For this review, take the finished solid that the model builds, in its own axes (mm). A direction names the side the tool comes from. Coordinates: 2 decimals unless noted, no trailing zeros. Write each loop counter-clockwise with the first axis right and the second up, starting at its lowest first coordinate (ties: lowest second). Pieces come first, ordered by that corner, then holes.
```python
from build123d import *

# Parameters (mm, degrees)
SKETCH1_W                    = 42.8625
SKETCH1_H                    = 44.27474
SKETCH1_R                    = 3
BASE_FLANGE1_DEPTH           = 3.175
EDGE_FLANGE1_STRIP_W         = 14.7
EDGE_FLANGE1_STRIP_H         = 3.175
EDGE_FLANGE1_STRIP_CUT_DEPTH = 44.27474
EDGE_FLANGE1_DEPTH           = 44.27474
CUT_EXTRUDE1_DEPTH           = 73.0427273
CUT_EXTRUDE1_DEPTH_BACK      = 3.175
M6_CLEARANCE_HOLE6_D         = 7


# Sheet-metal steps are written as plain solids
with BuildPart() as part:
    # Sketch1 → Base-Flange1 (new body)
    with BuildSketch(Plane.XY):
        Rectangle(SKETCH1_W, SKETCH1_H)
        with Locations((-0.79375, 3.26263)):
            Circle(SKETCH1_R, mode=Mode.SUBTRACT)
    extrude(amount=BASE_FLANGE1_DEPTH)

    # Edge-Flange1 strip (across the edge) → Edge-Flange1 strip cut (cut)
    with BuildSketch(Plane(origin=(-21.43125, 22.13737, 3.175), x_dir=(1, 0, 0), z_dir=(0, -1, 0))):
        with Locations((-6.35, -1.5875)):
            Rectangle(EDGE_FLANGE1_STRIP_W, EDGE_FLANGE1_STRIP_H)
    extrude(amount=EDGE_FLANGE1_STRIP_CUT_DEPTH, mode=Mode.SUBTRACT)

    # Edge-Flange1 section (across the edge) → Edge-Flange1 (add)
    with BuildSketch(Plane(origin=(-21.43125, 22.13737, 3.175), x_dir=(1, 0, 0), z_dir=(0, -1, 0))):
        with BuildLine():
            Line((-3.175, 1), (-3.175, 47.625))
            Line((-3.175, 47.625), (0, 47.625))
            Line((0, 47.625), (0, 1))
            ThreePointArc((0, 1), (0.292893219, 0.292893219), (1, 0))
            Line((1, 0), (1, -3.175))
            ThreePointArc((1, -3.175), (-1.952170811, -1.952170811), (-3.175, 1))
        make_face()
    extrude(amount=EDGE_FLANGE1_DEPTH)

    # Sketch10 → Cut-Extrude1 (cut, two sides: drawn at the far end of the back side and taken through both)
    with BuildSketch(Plane.ZY.offset(24.60625).offset(-CUT_EXTRUDE1_DEPTH_BACK)):
        Polygon((4.175, 22.13737), (50.8, -18.96237), (50.8, 22.13737), align=None)
    extrude(amount=CUT_EXTRUDE1_DEPTH + CUT_EXTRUDE1_DEPTH_BACK, mode=Mode.SUBTRACT)

    # M6 Clearance Hole6 (through all)
    with Locations(Plane.XY.offset(3.175)):
        with Locations((-0.79375, 3.26263)):
            Hole(M6_CLEARANCE_HOLE6_D / 2)


solid = part.part
```
1) Consider section C-C (z = 29). Give the boundary of the cut face in (x, y), then the cut area to 3 significant figures.
2) Tool access review of faces 1 (the face through (-22, -22.137, 14)), 2 (the face through (5, 0, 3.175)): name each direction out of +Z, -Z, +X, -X, +Y, -Y from which nothing blocks a thin tool from reaching the whole face with its end or side.
3) Clearance check with flat-ended pins moving along their axes: P1, Ø11, axis at x = -0.79, y = 3.26, coming from the -Z side; P2, Ø22, axis at y = -8.5, z = 27, coming from the +X side; P3, Ø6, axis at x = 5, y = -6.5, coming from the +Z side (3 decimals). State where each tip first meets the part, or that it passes through.
4) The part is to be moulded in two halves that separate along X. For faces 3 (the face through (-23.35, 0.31, 1.19)), 4 (the face through (-21.431, -10, 23)), 5 (the face through (-23, -21, 50.8)), 6 (the face through (-0.035, -0.154, 1.565)), say which applies: pulls with the +X half, pulls with the -X half, needs draft (parallel to the pull), parting line crosses it, or undercut.
5) Consider section D-D (y = -16). Give the boundary of the cut face in (x, z) (3 decimals), then the cut area to 3 significant figures.
6) Consider section A-A (y = -4.5). Give the boundary of the cut face in (x, z) (3 decimals).
7) For L1, parallel to Z at x = 0, y = 18.5 (3 decimals); L2, parallel to X at y = -19, z = 26; L3, parallel to Z at x = -21, y = 3.5, list the stretches that pass through material, from the lowest coordinate up.
8) Consider section B-B (x = -7). Give the boundary of the cut face in (y, z) (3 decimals), then the cut area to 3 significant figures.
Results:
1. outline: (-24.61, -22.14) - (-21.43, -22.14) - (-21.43, 0.25) - (-24.61, 0.25) - close
1. area: 71.1 mm2
2. face 1: +Z, -Z, +X, -X, -Y
2. face 2: +Z, +X, +Y, -Y
3. P1: stops at z = 0
3. P2: stops at x = -21.43
3. P3: stops at z = 3.175
4. face 3: pulls with the -X half
4. face 4: pulls with the +X half
4. face 5: needs draft
4. face 6: undercut
5. outline: (-24.606, 4.175) arc R4.175 ccw to (-20.431, 0) - (21.431, 0) - (21.431, 3.175) - (-20.431, 3.175) arc R1 cw to (-21.431, 4.175) - (-21.431, 47.439) - (-24.606, 47.439) - close
5. area: 283 mm2
6. outline: (-24.606, 4.175) arc R4.175 ccw to (-20.431, 0) - (21.431, 0) - (21.431, 3.175) - (-20.431, 3.175) arc R1 cw to (-21.431, 4.175) - (-21.431, 34.393) - (-24.606, 34.393) - close
7. L1: z = 0 to 3.175
7. L2: x = -24.61 to -21.43
7. L3: z = 0.04 to 3.35
8. outline: (-22.137, 0) - (22.137, 0) - (22.137, 3.175) - (-22.137, 3.175) - close
8. area: 141 mm2
